Geometry: final body of the model. Coordinates: model frame, mm. Coordinates: 2 decimals unless noted, no trailing zeros. Order: outer loops, then holes, each group sorted by start corner. A loop starts at its lowest first (then second) coordinate and runs counter-clockwise, first axis right, second up. Notation, with made-up numbers: (-28.75, 12.25) - (-9.75, 12.25) arc R20 cw to (-9.75, 50.25) - close; hole circle Ø11 at (77, 86). An arc over 180 degrees is marked (long way). Use one line per item in the form item = value. Start each with the question number.
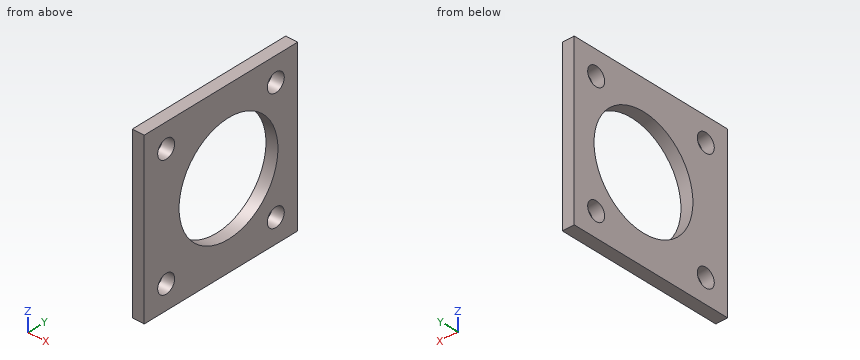
```python
from build123d import *

# Parameters (mm, degrees)
SKETCH1_W           = 44.45
SKETCH1_H           = 44.45
BOSS_EXTRUDE1_DEPTH = 3.175
SKETCH2_R           = 14.3129
SKETCH2_R_2         = 2.45745
CUT_EXTRUDE1_DEPTH  = 4.175


with BuildPart() as part:
    # Sketch1 → Boss-Extrude1 (new body)
    with BuildSketch(Plane(origin=(0, 0, 0), x_dir=(0, 0, -1), z_dir=(1, 0, 0))):
        Rectangle(SKETCH1_W, SKETCH1_H)
    extrude(amount=BOSS_EXTRUDE1_DEPTH)

    # Sketch2 → Cut-Extrude1 (cut, through all)
    with BuildSketch(Plane(origin=(3.175, 0, 0), x_dir=(0, 0, -1), z_dir=(1, 0, 0))):
        with Locations((0, 2.175)):
            Circle(SKETCH2_R)
        with Locations((-15.875, 15.875)):
            Circle(SKETCH2_R_2)
        with Locations((15.875, 15.875)):
            Circle(SKETCH2_R_2)
        with Locations((15.875, -15.875)):
            Circle(SKETCH2_R_2)
        with Locations((-15.875, -15.875)):
            Circle(SKETCH2_R_2)
    extrude(amount=-CUT_EXTRUDE1_DEPTH, mode=Mode.SUBTRACT)


solid = part.part
```
(1) Cut plane B-B on y = 1.5. Return the cut outline in (x, z) (3 decimals).
(2) Cut plane D-D on x = 0.9. Return the cut outline in (y, z) (3 decimals), plus the area to 3 significant figures.
(3) Material intervals for L1, parallel to Z at x = 0.25, y = -14.5 (3 decimals); L2, parallel to Y at x = 1.45, z = 15 (3 decimals); L3, parallel to Z at x = 2.8, y = 2 (3 decimals), sorted ascending. Write a range as from..to.
(4) Cut plane C-C on z = 15.5. Return the cut outline in (x, y) (3 decimals).
(5) Cut plane A-A on z = 0. Return the cut outline in (x, y) (3 decimals), plus the area to 3 significant figures.
Check sheet entries:
q1.outline = (0, -22.225) - (3.175, -22.225) - (3.175, -14.297) - (0, -14.297) - close; (0, 14.297) - (3.175, 14.297) - (3.175, 22.225) - (0, 22.225) - close
q2.outline = (-22.225, -22.225) - (22.225, -22.225) - (22.225, 22.225) - (-22.225, 22.225) - close; hole circle Ø4.915 at (-15.875, -15.875); hole circle Ø4.915 at (-15.875, 15.875); hole circle Ø28.626 at (2.175, 0); hole circle Ø4.915 at (15.875, -15.875); hole circle Ø4.915 at (15.875, 15.875)
q2.area = 1,260 mm^2
q3.L1 = -22.225..-17.912, -13.838..13.838, 17.912..22.225
q3.L2 = -22.225..-18.171, -13.579..13.579, 18.171..22.225
q3.L3 = -22.225..-14.312, 14.312..22.225
q4.outline = (0, -22.225) - (3.175, -22.225) - (3.175, -18.304) - (0, -18.304) - close; (0, -13.446) - (3.175, -13.446) - (3.175, 13.446) - (0, 13.446) - close; (0, 18.304) - (3.175, 18.304) - (3.175, 22.225) - (0, 22.225) - close
q5.outline = (0, -22.225) - (3.175, -22.225) - (3.175, -12.138) - (0, -12.138) - close; (0, 16.488) - (3.175, 16.488) - (3.175, 22.225) - (0, 22.225) - close
q5.area = 50.2 mm^2
